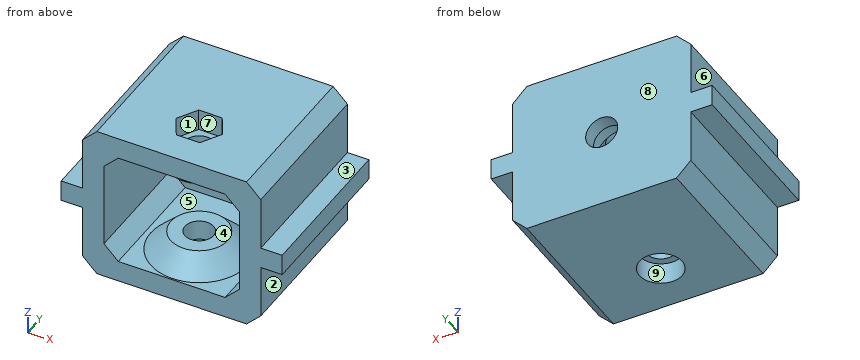
from build123d import *

# Parameters (mm, degrees)
SKETCH1_W           = 25
SKETCH1_H           = 22
BOSS_EXTRUDE1_DEPTH = 22
SKETCH3_W           = 31
SKETCH3_H           = 3
BOSS_EXTRUDE2_DEPTH = 22
SKETCH4_W           = 19
SKETCH4_H           = 16
CUT_EXTRUDE3_DEPTH  = 17
SKETCH5_R           = 3
BOSS_EXTRUDE3_DEPTH = 2.8
BOSS_EXTRUDE4_START = 2.8
SKETCH6_R           = 3
BOSS_EXTRUDE4_DEPTH = 2.8
SKETCH7_R           = 2
CUT_EXTRUDE4_DEPTH  = 35.759890679
CHAMFER1_SIZE       = 3.8
SKETCH8_R           = 3
CUT_EXTRUDE5_DEPTH  = 3
CUT_EXTRUDE6_DEPTH  = 3
CHAMFER2_SIZE       = 2
SKETCH10_R          = 3.75
CUT_EXTRUDE7_DEPTH  = 3
SKETCH11_R          = 2.25
CUT_EXTRUDE8_DEPTH  = 28.590759323


with BuildPart() as part:
    # Sketch1 → Boss-Extrude1 (new body)
    with BuildSketch(Plane(origin=(0, 0, 0), x_dir=(1, 0, 0), z_dir=(0, 1, 0))):
        Rectangle(SKETCH1_W, SKETCH1_H)
    extrude(amount=BOSS_EXTRUDE1_DEPTH)

    # Sketch3 → Boss-Extrude2 (add)
    with BuildSketch(Plane(origin=(0, 0, 0), x_dir=(1, 0, 0), z_dir=(0, 1, 0))):
        Rectangle(SKETCH3_W, SKETCH3_H)
    extrude(amount=BOSS_EXTRUDE2_DEPTH)

    # Sketch4 → Cut-Extrude3 (cut)
    with BuildSketch(Plane(origin=(0, 0, 0), x_dir=(1, 0, 0), z_dir=(0, 1, 0))):
        Rectangle(SKETCH4_W, SKETCH4_H)
    extrude(amount=CUT_EXTRUDE3_DEPTH, mode=Mode.SUBTRACT)

    # Sketch5 → Boss-Extrude3 (add)
    with BuildSketch(Plane(origin=(0, 0, -8), x_dir=(-1, 0, 0), z_dir=(0, 0, -1))):
        with Locations((0, 7)):
            Circle(SKETCH5_R)
    extrude(amount=-BOSS_EXTRUDE3_DEPTH)

    # Sketch6 → Boss-Extrude4 (add)
    with BuildSketch(Plane(origin=(0, 0, 8), x_dir=(-1, 0, 0), z_dir=(0, 0, -1)).offset(BOSS_EXTRUDE4_START)):
        with Locations((0, 7)):
            Circle(SKETCH6_R)
    extrude(amount=-BOSS_EXTRUDE4_DEPTH)

    # Sketch7 → Cut-Extrude4 (cut, through all)
    with BuildSketch(Plane(origin=(0, 0, -11), x_dir=(-1, 0, 0), z_dir=(0, 0, -1))):
        with Locations((0, 7)):
            Circle(SKETCH7_R)
    extrude(amount=-CUT_EXTRUDE4_DEPTH, mode=Mode.SUBTRACT)

    # Chamfer1
    # the kernel refuses this chamfer: 3.8 mm, written as the material it adds along each edge
    with BuildSketch(Plane(origin=(0, 7, 8), x_dir=(-1, 0, 0), z_dir=(0, -1, 0))) as chamfer1_piece_1_section:
        Polygon((3 + CHAMFER1_SIZE, 0), (3, CHAMFER1_SIZE), (3, 0), align=None)
    chamfer1_piece_1 = revolve(axis=Axis((0, 7, 8), (0, 0, -1)), mode=Mode.PRIVATE)
    chamfer1_piece_1 = split(chamfer1_piece_1, bisect_by=Plane(origin=(5.412454592, 7, 5.2), z_dir=(0, 0, 1)), keep=Keep.TOP, mode=Mode.PRIVATE)
    add(chamfer1_piece_1)
    with BuildSketch(Plane(origin=(0, 7, -8), x_dir=(-1, 0, 0), z_dir=(0, -1, 0))) as chamfer1_piece_2_section:
        Polygon((3 + CHAMFER1_SIZE, 0), (3, -CHAMFER1_SIZE), (3, 0), align=None)
    chamfer1_piece_2 = revolve(axis=Axis((0, 7, -8), (0, 0, -1)), mode=Mode.PRIVATE)
    chamfer1_piece_2 = split(chamfer1_piece_2, bisect_by=Plane(origin=(5.412454592, 7, -5.2), z_dir=(0, 0, -1)), keep=Keep.TOP, mode=Mode.PRIVATE)
    add(chamfer1_piece_2)

    # Sketch8 → Cut-Extrude5 (cut)
    with BuildSketch(Plane(origin=(0, 0, -11), x_dir=(-1, 0, 0), z_dir=(0, 0, -1))):
        with Locations((0, 7)):
            Circle(SKETCH8_R)
    extrude(amount=-CUT_EXTRUDE5_DEPTH, mode=Mode.SUBTRACT)

    # Sketch9 → Cut-Extrude6 (cut)
    with BuildSketch(Plane.XY.offset(11)):
        Polygon((1.645448267, 9.85), (-1.645448267, 9.85), (-3.290896534, 7), (-1.645448267, 4.15), (1.645448267, 4.15), (3.290896534, 7), align=None)
    extrude(amount=-CUT_EXTRUDE6_DEPTH, mode=Mode.SUBTRACT)

    # Chamfer2
    chamfer2_edges = [part.edges().sort_by_distance(p)[0] for p in [
        (-9.5, 8.5, 8),
        (-9.5, 8.5, -8),
        (9.5, 8.5, -8),
        (9.5, 8.5, 8),
        (12.5, 11, 11),
        (-12.5, 11, 11),
        (-12.5, 11, -11),
        (12.5, 11, -11),
    ]]
    chamfer(chamfer2_edges, length=CHAMFER2_SIZE)

    # Sketch10 → Cut-Extrude7 (cut)
    with BuildSketch(Plane.XZ.offset(-17)):
        with Locations(Location((0, 0, 0), (0, 0, 270))):
            Circle(SKETCH10_R)
    extrude(amount=-CUT_EXTRUDE7_DEPTH, mode=Mode.SUBTRACT)

    # Sketch11 → Cut-Extrude8 (cut, through all)
    with BuildSketch(Plane.XZ.offset(-20)):
        with Locations(Location((0, 0, 0), (0, 0, 270))):
            Circle(SKETCH11_R)
    extrude(amount=-CUT_EXTRUDE8_DEPTH, mode=Mode.SUBTRACT)


solid = part.part
Input: part model. Units: mm. Frame: model coordinates. Face numbers are marked on the shaded views. A direction names the side the tool comes from. Coordinates: 2 decimals unless noted, no trailing zeros. Loops run counter-clockwise (first coordinate to the right, second up) from the corner with the lowest first, then second, coordinate; pieces in that order, holes last. Notation, with made-up numbers: (-5.75, -18) - (41.25, -18) arc R27 cw to (41.25, -1) - close; hole circle Ø11 at (47.5, 80). An arc over 180 degrees is marked (long way). Answer in a Markdown table with one row per item. Add a question column.
Item 1: Section query C-C on x = -9. Return the cut outline in (y, z).
Item 2: Section query A-A on z = 7. Return the cut outline in (x, y).
Item 3: Contact query for flat-ended pins moving along their axis: P1, Ø6, axis at x = 0, z = 0, coming from the -Y side; P2, Ø2, axis at y = 17, z = -4.5, coming from the +X side; P3, Ø6, axis at y = 14, z = -5, coming from the -X side; P4, Ø1.7, axis at x = -1, y = 7, coming from the +Z side. Output: stop coordinate, or through.
Item 4: Section query D-D on z = -4.75. Return the cut outline in (x, y).
Item 5: Section query B-B on z = 0. Return the cut outline in (x, y).
Item 6: Mould query, pull axis Y, two halves, no side actions, for the marked faces 6, 7, 8 and 9. Classes: released by +Y, released by -Y, zero draft, split by the parting line, or undercut.
Item 7: Access query for the marked faces 1, 2, 3, 4 and 5. Directions: +Z, -Z, +X, -X, +Y, -Y. A direction counts if a zero-diameter tool reaches every point of the face in a straight line with its end or side. Return the directions, or none.
Item 8: Line query: line 1 along Z through (x, y) = (2, 4.5); line 2 along X through (y, z) = (13.5, 0.5); line 3 along X through (y, z) = (18.4, 0). Output: solid intervals per line, ascending. Write a range as [from, to].
Recorded:
| question | item | result |
|---|---|---|
| 1 | outline | (0, -11) - (22, -11) - (22, 11) - (0, 11) - (0, 6.5) - (17, 6.5) - (17, -6.5) - (0, -6.5) - close |
| 2 | outline | (-12.5, 0) - (-8.5, 0) - (-8.5, 17) - (8.5, 17) - (8.5, 0) - (12.5, 0) - (12.5, 22) - (-12.5, 22) - close; circle Ø11.6 at (0, 7); hole circle Ø4 at (0, 7) |
| 3 | P1 | y = 20 |
| 3 | P2 | x = 12.5 |
| 3 | P3 | x = -12.5 |
| 3 | P4 | through |
| 4 | outline | (-12.5, 0) - (-9.5, 0) - (-9.5, 17) - (9.5, 17) - (9.5, 0) - (12.5, 0) - (12.5, 22) - (-12.5, 22) - close |
| 5 | outline | (-15.5, 0) - (-9.5, 0) - (-9.5, 17) - (-3.75, 17) - (-3.75, 20) - (-2.25, 20) - (-2.25, 22) - (-15.5, 22) - close; (2.25, 20) - (3.75, 20) - (3.75, 17) - (9.5, 17) - (9.5, 0) - (15.5, 0) - (15.5, 22) - (2.25, 22) - close |
| 6 | face 6 | zero draft |
| 6 | face 7 | undercut |
| 6 | face 8 | released by +Y |
| 6 | face 9 | undercut |
| 7 | face 1 | +Z |
| 7 | face 2 | -Z, +X, +Y, -Y |
| 7 | face 3 | +Z, +X, +Y, -Y |
| 7 | face 4 | -Y |
| 7 | face 5 | none |
| 8 | line 1 | [-11, -5.2], [5.2, 11] |
| 8 | line 2 | [-15.5, -9.5], [9.5, 15.5] |
| 8 | line 3 | [-15.5, -3.75], [3.75, 15.5] |
